Build history of the part. All positions in model axes, mm. Round coordinates to 2 decimals unless told otherwise and drop trailing zeros. Write each loop counter-clockwise with the first axis right and the second up, starting at its lowest first coordinate (ties: lowest second). Pieces come first, ordered by that corner, then holes. Notation, with made-up numbers: (17.25, 36.5) -> (22.25, 36.5) arc R37 ccw to (22.25, 74.5) -> close; hole circle Ø10 at (34.5, 22). An arc over 180 degrees is marked (long way). Answer in a Markdown table with one row per item.
```python
from build123d import *

# Parameters (mm, degrees)
SKETCH_1_R               = 13
SKETCH_1_R_2             = 11
EXTRUDE_1_DEPTH          = 6
SKETCH_2_R               = 0.75
CUT_EXTRUDE_1_DEPTH      = 14
PATTERN_CIRCULAR_1_COUNT = 16
SKETCH_3_W               = 36.79853237
SKETCH_3_H               = 11.94610836
CUT_EXTRUDE_2_DEPTH      = 14.0000001


with BuildPart() as part:
    # ｽｹｯﾁ1 → ﾎﾞｽ - 押し出し1 (new body)
    with BuildSketch(Plane.XY):
        Circle(SKETCH_1_R)
        Circle(SKETCH_1_R_2, mode=Mode.SUBTRACT)
    extrude(amount=EXTRUDE_1_DEPTH)

    # ｽｹｯﾁ2 → ｶｯﾄ - 押し出し1 (cut, through all)
    with BuildSketch(Plane(origin=(0, 0, 0), x_dir=(1, 0, 0), z_dir=(0, 1, 0))):
        with Locations((0, -3)):
            Circle(SKETCH_2_R)
    cut_extrude_1 = extrude(amount=-CUT_EXTRUDE_1_DEPTH, mode=Mode.SUBTRACT)

    # 円形ﾊﾟﾀｰﾝ1: ｶｯﾄ - 押し出し1 ×16 about axis
    pattern_circular_1_axis = Axis((0, 0, 0), (0, 0, 1))
    for i in range(1, PATTERN_CIRCULAR_1_COUNT):
        add(cut_extrude_1.rotate(pattern_circular_1_axis, i * 360 / PATTERN_CIRCULAR_1_COUNT), mode=Mode.SUBTRACT)

    # ｽｹｯﾁ3 → ｶｯﾄ - 押し出し2 (cut, through all)
    with BuildSketch(Plane(origin=(0, 0, 0), x_dir=(1, 0, 0), z_dir=(0, 1, 0))):
        with Locations((0, -2.028241391)):
            Rectangle(SKETCH_3_W, SKETCH_3_H)
    extrude(amount=-CUT_EXTRUDE_2_DEPTH, mode=Mode.SUBTRACT)


solid = part.part
```
Q1. Drop flat-ended pins along their axis: P1, Ø3, axis at x = 4.5, y = 8, coming from the +Z side; P2, Ø2.5, axis at x = 0, z = 3, coming from the -Y side; P3, Ø3, axis at x = -3.5, z = 4.5, coming from the +Y side; P4, Ø1, axis at x = -1, z = 4.5, coming from the +Y side. Give the stop position or say it passes through.
A:
| item | result |
|---|---|
| P1 | through |
| P2 | y = 10.93 |
| P3 | y = 12.85 |
| P4 | y = 12.99 |
Q2. Two-plate mould, pull along Y, no slides. Class faces 1 (the cylindrical face through (5.132, 10.834, 3.456)), 2 (the flat face through (2, 11, 6)), 3 (the flat face through (-12, 0, 5)): released by +Y, released by -Y, zero draft, split by the parting line, or undercut.
A:
| item | result |
|---|---|
| face 1 | undercut |
| face 2 | zero draft |
| face 3 | released by -Y |
Q3. Saw through at A-A on x = 0. Write the cut outline in (y, z).
A:
| item | result |
|---|---|
| outline | (11, 0) -> (13, 0) -> (13, 2.25) -> (11, 2.25) -> close; (11, 3.75) -> (13, 3.75) -> (13, 6) -> (11, 6) -> close |
Q4. Saw through at B-B on z = 3. State how many separate pieces and enclosed holes the cut face has, plus the area to 3 significant figures.
A:
| item | result |
|---|---|
| separate pieces | 8 |
| enclosed holes | 0 |
| area | 51.4 mm² |
Q5. Saw through at D-D on z = 0.5. Write the cut outline in (x, y), plus the area to 3 significant figures.
A:
| item | result |
|---|---|
| outline | (-13, 0) -> (-11, 0) arc R11 cw to (11, 0) -> (13, 0) arc R13 ccw to start |
| area | 75.4 mm² |
Q6. Saw through at C-C on y = 6.5. Write the cut outline in (x, z), plus the area to 3 significant figures.
A:
| item | result |
|---|---|
| outline | (-11.26, 0) -> (-8.87, 0) -> (-8.87, 6) -> (-11.26, 6) -> close; (8.87, 0) -> (11.26, 0) -> (11.26, 6) -> (8.87, 6) -> close |
| area | 28.6 mm² |
Q7. Wall check: line 1 (Z direction, x = 0, y = 11.45); line 2 (X direction, y = 11.5, z = 2.75); line 3 (X direction, y = 11.55, z = 3). Give the ranges that are in metal, low to high. Write a range as [from, to].
A:
| item | result |
|---|---|
| line 1 | [0, 2.25], [3.75, 6] |
| line 2 | [-6.06, -5.53], [-4, -0.71], [0.71, 4], [5.53, 6.06] |
| line 3 | [-5.97, -5.6], [-3.97, -0.75], [0.75, 3.97], [5.6, 5.97] |
